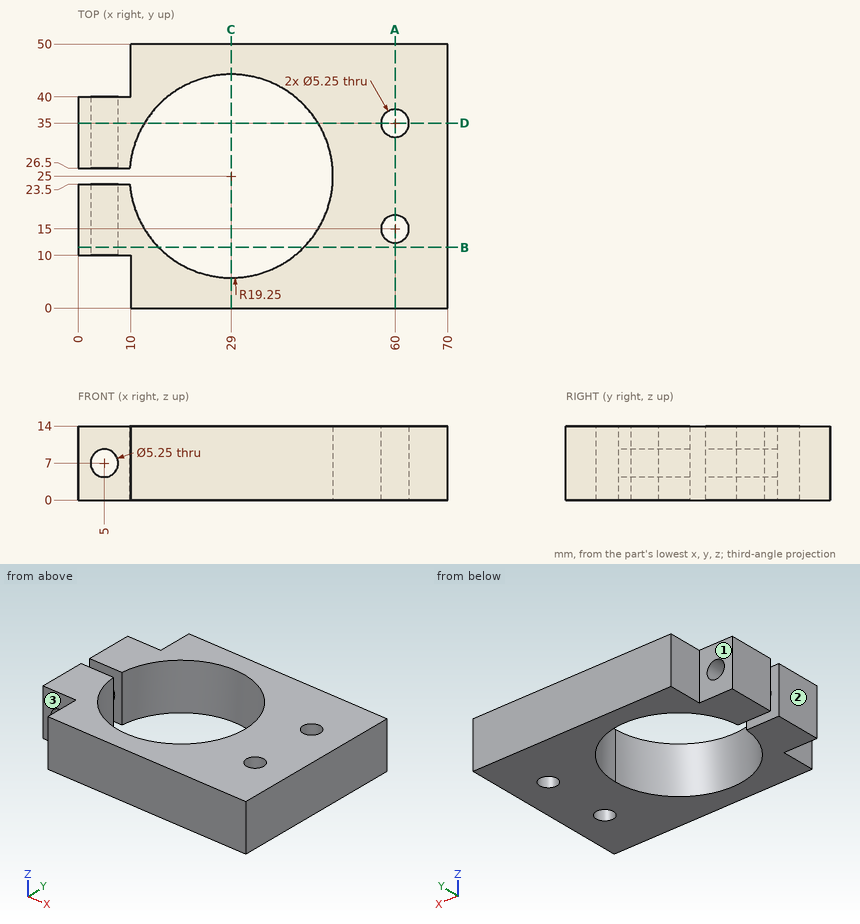
The figure shows three views and two pictorial views of one solid part (mm, origin at its lowest corner). Answer the questions. A direction names the side the tool comes from. Round coordinates to 2 decimals unless told otherwise and drop trailing zeros. Write each loop counter-clockwise with the first axis right and the second up, starting at its lowest first coordinate (ties: lowest second). Pieces come first, ordered by that corner, then holes. Notation, with made-up numbers: M 53.25,23.25 L 80.25,23.25 A13 cw 80.25,35.25 Z; hole C 80.5,1.25 d2. An arc over 180 degrees is marked long. Use a Markdown table: item, result.
1) The part is cut by section B-B (y = 11.5). Write down the section's boundary in (x, z) (3 decimals), plus the area to 3 significant figures.
Answers follow:
| item | result |
|---|---|
| outline | M 0,0 L 15.277,0 L 15.277,14 L 0,14 Z; M 42.723,0 L 70,0 L 70,14 L 42.723,14 Z; hole C 5,7 d5.25 |
| area | 574 mm2 |
2) The part is cut by section D-D (y = 35). Write down the section's boundary in (x, z) (3 decimals), plus the area to 3 significant figures.
Answers follow:
| item | result |
|---|---|
| outline | M 0,0 L 12.551,0 L 12.551,14 L 0,14 Z; M 45.449,0 L 57.375,0 L 57.375,14 L 45.449,14 Z; M 62.625,0 L 70,0 L 70,14 L 62.625,14 Z; hole C 5,7 d5.25 |
| area | 424 mm2 |
3) The part is cut by section A-A (x = 60). Write down the section's boundary in (y, z) (3 decimals).
Answers follow:
| item | result |
|---|---|
| outline | M 0,0 L 12.375,0 L 12.375,14 L 0,14 Z; M 17.625,0 L 32.375,0 L 32.375,14 L 17.625,14 Z; M 37.625,0 L 50,0 L 50,14 L 37.625,14 Z |
4) A tool of negligible diameter and unlimited length cuts with its end or side. For the marked faces 1, 2 and 3, from which of +Z, -Z, +X, -X, +Y, -Y can it reach the whole face along a straight path? Write none if from no direction.
Answers follow:
| item | result |
|---|---|
| face 1 | +Z, -Z, -X, +Y |
| face 2 | +Z, -Z, -X, +Y, -Y |
| face 3 | +Z, -Z, -X, -Y |
5) Flat-ended cylindrical pins translate along their axes: pin 1 (3 mm diameter, centred on x = 6.5, z = 10, fed in from +Y); pin 2 (8 mm diameter, centred on x = 3, z = 7.5, fed in from -Y). Find the tip coordinate at first contact, or state that the pin passes through.
Answers follow:
| item | result |
|---|---|
| pin 1 | stops at y = 40 |
| pin 2 | stops at y = 10 |
6) Straight lines are drawn through the part: line 1 along Y through (x, z) = (60, 3.75) (3 decimals); line 2 along Y through (x, z) = (28.5, 1.75); line 3 along X through (y, z) = (34, 9). For each, find the intervals that lie inside material, in ascending order. Write a range as [from, to].
Answers follow:
| item | result |
|---|---|
| line 1 | y = [0, 12.375], [17.625, 32.375], [37.625, 50] |
| line 2 | y = [0, 5.76], [44.24, 50] |
| line 3 | x = [0, 3.3], [6.7, 11.98], [46.02, 57.57], [62.43, 70] |
7) The part is cut by section C-C (x = 29). Write down the section's boundary in (y, z).
Answers follow:
| item | result |
|---|---|
| outline | M 0,0 L 5.75,0 L 5.75,14 L 0,14 Z; M 44.25,0 L 50,0 L 50,14 L 44.25,14 Z |
